Autodesk Inventor part; units mm, degrees
ref_plane "XZ Plane" through (0, 0, 0) normal (0, 1, 0) x (-1, 0, 0)
ref_plane "XY Plane" through (0, 0, 0) normal (0, 0, 1) x (1, 0, 0)
sketch "Эскиз1" plane through (0, 0, 0) normal (0, 0, 1) x (1, 0, 0)
  circle A0 centre (0, 0) radius 45.15
  circle A1 centre (0, 0) radius 46.75
  dimension "d0" = 90.3
  dimension "d1" = 93.5
extrude "Выдавливание1" add sketch "Эскиз1" along normal blind 160
fillet "Сопряжение1" radius 0.8 4 edges at (-46.75, 0, 160) (-45.15, 0, 160) (-46.75, 0, 0) (-45.15, 0, 0)
sketch "Эскиз2" plane through (0, 0, 0) normal (1, 0, 0) x (0, 1, 0)
  circle A0 centre (0, 15) radius 2
  circle A1 centre (0, 145) radius 2
  point P0 (0, 0)
  dimension "d5" = 4
  dimension "d6" = 4
  dimension "d7" = 15
  dimension "d8" = 145
hole "Отверстие1" at (0, 0, 145) at (0, 0, 15) direction (-1, 0, 0) diameter 4 end through all both
equation "\"d0\" = dInternal"
equation "\"d1\" = dInternal + wallThickness"
equation "\"d2\" = tubeHeight"
equation "\"d4\" = 0.25 * wallThickness"
equation "\"d5\" = dHole"
equation "\"d6\" = dHole"
equation "\"d9\" = dHole"
equation "\"dInternal\" = 90.3"
equation "\"wallThickness\" = 3.2"
equation "\"tubeHeight\" = 160"
equation "\"dHole\" = 4"
equation "\"distanceHoles\" = 15"
properties part number "EimarTube"
Model file for the job. Use its own axes, mm. Coordinates: 2 decimals unless noted, no trailing zeros. Write each loop counter-clockwise with the first axis right and the second up, starting at its lowest first coordinate (ties: lowest second). Pieces come first, ordered by that corner, then holes. Notation, with made-up numbers: (42, -26) - (75, -26) arc R32 cw to (75, 4) - close; hole circle Ø10 at (86.25, 63.5). An arc over 180 degrees is marked (long way). One line per item, written item: value. Start each with the question number.
1. Mould opens along Y. For faces 1 (the cylindrical face through (25.13, -39.42, 78.89)), 2 (the cylindrical face through (-9.788, 44.076, 78.891)) say: released by +Y, released by -Y, zero draft, split by the parting line, or undercut.
2. Slice it at B-B (y = 0). Count the separate pieces of the cut face and the enclosed holes in it, plus the area to 3 significant figures.
3. Slice it at D-D (z = 81). Write the cut outline in (x, y).
4. Slice it at C-C (z = 145). Write the cut outline in (x, y).
5. Probe line 1 (Y direction, x = 0, z = 104.5); line 2 (Z direction, x = 46, y = 0); line 3 (Z direction, x = 45.4, y = 0). List the from-to ranges inside material, lowest first. Write a range as from..to.
6. Flat gauge pins, fed straight in: pin 1 (2 mm diameter, centred on x = -17.5, z = 133.5, fed in from +Y); pin 2 (3.5 mm diameter, centred on y = 0, z = 145, fed in from -X); pin 3 (8 mm diameter, centred on x = -32.5, z = 105, fed in from -Y); pin 4 (10 mm diameter, centred on y = 23, z = 74, fed in from +X). Where does each tip first touch, or does it go through?
Answers below:
1. face 1: split by the parting line
1. face 2: undercut
2. separate pieces: 6
2. enclosed holes: 0
2. area: 485 mm^2
3. outline: circle Ø93.5 at (0, 0); hole circle Ø90.3 at (0, 0)
4. outline: (-46.71, -2) arc R46.75 ccw to (46.71, -2) - (45.11, -2) arc R45.15 cw to (-45.11, -2) - close; (-46.71, 2) - (-45.11, 2) arc R45.15 cw to (45.11, 2) - (46.71, 2) arc R46.75 ccw to start
5. line 1: y = -46.75..-45.15, 45.15..46.75
5. line 2: z = 0..13, 17..143, 147..160
5. line 3: z = 0.22..13, 17..143, 147..159.78
6. pin 1: stops at y = 43.74
6. pin 2: passes through
6. pin 3: stops at y = -37.06
6. pin 4: stops at x = 43.15
